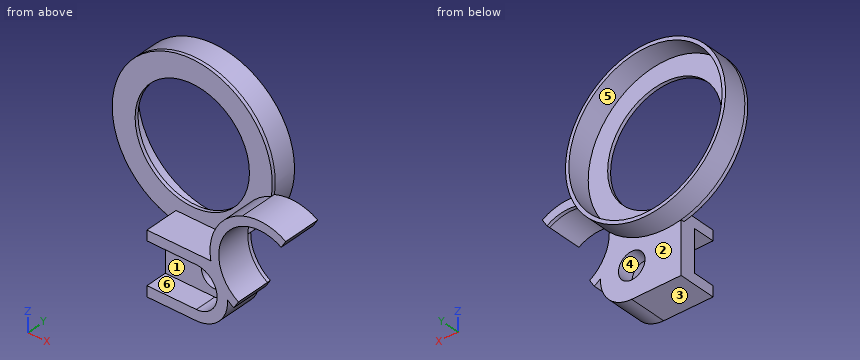
```python
from build123d import *

# Parameters (mm, degrees)
SKETCH1_R           = 50
SKETCH1_R_2         = 11.615083761
BOSS_EXTRUDE1_DEPTH = 3
SKETCH2_R           = 70
SKETCH2_R_2         = 67
BOSS_EXTRUDE3_DEPTH = 20
SKETCH4_R           = 11.615083761
BOSS_EXTRUDE6_DEPTH = 30
CUT_EXTRUDE2_DEPTH  = 19


with BuildPart() as part:
    # Sketch1 → Boss-Extrude1 (new body)
    with BuildSketch(Plane(origin=(0, 0, 0), x_dir=(1, 0, 0), z_dir=(0, 1, 0))):
        with BuildLine():
            Line((61.670303131, 88.507050428), (65.738918694, 82.002662996))
            ThreePointArc((65.738918694, 82.002662996), (52.910005118, 68.514839013), (48.562558373, 50.415056524))
            ThreePointArc((48.562558373, 50.415056524), (59.803165171, 36.381058747), (67.097930635, 19.94662138))
            ThreePointArc((67.097930635, 19.94662138), (85.226692334, 15.486926368), (103.142834496, 20.735995847))
            Line((103.142834496, 20.735995847), (107.211450059, 14.231608415))
            ThreePointArc((107.211450059, 14.231608415), (88.628926733, 8.008407228), (69.198869979, 10.560132275))
            ThreePointArc((69.198869979, 10.560132275), (-39.949778038, -57.480563973), (-14.223379462, 68.539736479))
            Line((-14.223379462, 68.539736479), (-14.223379462, 113.780543001))
            Line((-14.223379462, 113.780543001), (28.94098919, 113.780543001))
            ThreePointArc((28.94098919, 113.780543001), (48.93114235, 105.106024988), (56.25040353, 84.580872081))
            ThreePointArc((56.25040353, 84.580872081), (58.884844334, 86.648197778), (61.670303131, 88.507050428))
        make_face()
        Circle(SKETCH1_R, mode=Mode.SUBTRACT)
        with Locations((28.94098919, 86.409945266)):
            Circle(SKETCH1_R_2, mode=Mode.SUBTRACT)
    extrude(amount=BOSS_EXTRUDE1_DEPTH)

    # Sketch2 → Boss-Extrude3 (add)
    with BuildSketch(Plane(origin=(0, 3, 0), x_dir=(1, 0, 0), z_dir=(0, 1, 0))):
        Circle(SKETCH2_R)
        Circle(SKETCH2_R_2, mode=Mode.SUBTRACT)
    extrude(amount=BOSS_EXTRUDE3_DEPTH)

    # Sketch4 → Boss-Extrude6 (add)
    with BuildSketch(Plane.XZ):
        with BuildLine():
            Line((107.211450059, -14.231608415), (103.142834496, -20.735995847))
            ThreePointArc((103.142834496, -20.735995847), (53.80754302, -32.66737152), (65.738918694, -82.002662996))
            Line((65.738918694, -82.002662996), (61.670303131, -88.507050428))
            ThreePointArc((61.670303131, -88.507050428), (58.884844334, -86.648197778), (56.25040353, -84.580872081))
            ThreePointArc((56.25040353, -84.580872081), (48.93114235, -105.106024988), (28.94098919, -113.780543001))
            Line((28.94098919, -113.780543001), (-14.223379462, -113.780543001))
            Line((-14.223379462, -113.780543001), (-14.223379462, -59.37804429))
            Line((-14.223379462, -59.37804429), (41.620673144, -59.37804429))
            ThreePointArc((41.620673144, -59.37804429), (46.511966871, -29.942543741), (69.198869979, -10.560132275))
            ThreePointArc((69.198869979, -10.560132275), (88.628926733, -8.008407228), (107.211450059, -14.231608415))
        make_face()
        with Locations((28.94098919, -86.409945266)):
            Circle(SKETCH4_R, mode=Mode.SUBTRACT)
    extrude(amount=BOSS_EXTRUDE6_DEPTH)

    # Sketch6 → Cut-Extrude2 (cut)
    with BuildSketch(Plane.XZ.offset(30)):
        with BuildLine():
            Line((28.94098919, -104.597730163), (-14.223379462, -104.597730163))
            Line((-14.223379462, -104.597730163), (-14.223379462, -68.222160369))
            Line((-14.223379462, -68.222160369), (28.94098919, -68.222160369))
            ThreePointArc((28.94098919, -68.222160369), (47.128774087, -86.409945266), (28.94098919, -104.597730163))
        make_face()
    extrude(amount=-CUT_EXTRUDE2_DEPTH, mode=Mode.SUBTRACT)


solid = part.part
```
Part model, mm, in its own coordinate system. Face numbers are marked on the shaded views. A direction names the side the tool comes from. Round coordinates to 2 decimals unless told otherwise and drop trailing zeros. Order: outer loops, then holes, each group sorted by start corner. A loop starts at its lowest first (then second) coordinate and runs counter-clockwise, first axis right, second up. Notation, with made-up numbers: M 83,74.25 L 112,74.25 A13 cw 112,80.25 Z; hole C 11.25,76.25 d4. An arc over 180 degrees is marked long. Answer in a Markdown table with one row per item. Add a question column.
Q1. Cut at B-B on z = 0. Give the cut face in (x, y).
Q2. Wall check: L1, parallel to Z at x = 0, y = 1.05; L2, parallel to X at y = 16.75, z = 0. Give the ranges that are in metal, low to high. Write a range as from..to.
Q3. 3-axis set-ups, long thin cutter, end or side, ignore diameter. For the marked faces 4, 5 and 6: which of +Z, -Z, +X, -X, +Y, -Y reach the whole face in a straight line?
Q4. Cut at A-A on x = 0. Give the cut face in (y, z).
Q5. Pin check, flat tips, straight feed: pin 1 (16.5 mm diameter, centred on y = -11, z = -97.5, fed in from -X); pin 2 (4 mm diameter, centred on x = 91.5, z = -16.5, fed in from +Y); pin 3 (12 mm diameter, centred on y = -12, z = -1.5, fed in from +X); pin 4 (21 mm diameter, centred on x = 1.5, y = -23.5, fed in from +Z). Stop position of each tip, or through.
Q6. Mould opens along Z. For the marked faces 1, 2 and 3 say: +Z half, -Z half, draft (parallel to the pull), parting line (faces both ways), or undercut.
Established:
| question | item | result |
|---|---|---|
| 1 | outline | M -70,0 L -50,0 L -50,3 L -67,3 L -67,23 L -70,23 Z; M 50,0 L 70,0 L 70,23 L 67,23 L 67,3 L 50,3 Z |
| 2 | L1 | z = -113.78..-50, 50..70 |
| 2 | L2 | x = -70..-67, 67..70 |
| 3 | face 4 | +Y, -Y |
| 3 | face 5 | +Y |
| 3 | face 6 | -X, -Y |
| 4 | outline | M -30,-113.78 L 3,-113.78 L 3,-70 L 23,-70 L 23,-67 L 3,-67 L 3,-50 L 0,-50 L 0,-59.38 L -30,-59.38 L -30,-68.22 L -11,-68.22 L -11,-104.6 L -30,-104.6 Z; M 0,50 L 3,50 L 3,67 L 23,67 L 23,70 L 0,70 Z |
| 5 | pin 1 | stops at x = -14.22 |
| 5 | pin 2 | stops at y = 3 |
| 5 | pin 3 | passes through |
| 5 | pin 4 | stops at z = -59.38 |
| 6 | face 1 | undercut |
| 6 | face 2 | draft |
| 6 | face 3 | -Z half |
